from build123d import *

# Parameters (mm, degrees)
F1_DEPTH  = 8
F3_W      = 8
F3_H      = 8
F3_R      = 2.4
F4_DEPTH  = 1.7
F5_R      = 2.4
F6_DEPTH  = 1.7
F9_R      = 2.4
F10_DEPTH = 25.4


with BuildPart() as f1:
    # F0 (on Front) → F1 (new body)
    with BuildSketch(Plane.XZ):
        Polygon((-2.4, 9.6), (-4, 9.6), (-4, 0), (4, 0), (4, 9.6), (2.4, 9.6), (2.4, 11.3), (-2.4, 11.3), align=None)
    extrude(amount=F1_DEPTH)

    # F3 (on plane+point) → F4 (cut, through all)
    with BuildSketch(Plane.XY.offset(11.3)):
        with Locations((0, -4)):
            Rectangle(F3_W, F3_H)
        with Locations((0, -4)):
            Circle(F3_R, mode=Mode.SUBTRACT)
    extrude(amount=-F4_DEPTH, mode=Mode.SUBTRACT)

    # F5 (on Top) → F6 (cut)
    with BuildSketch(Plane.XY):
        with Locations((0, -4)):
            Circle(F5_R)
    extrude(amount=F6_DEPTH, mode=Mode.SUBTRACT)

    # F8: F1 across plane


with BuildPart() as f1_1:
    add(f1.part)
    add(f1.part.mirror(Plane.YZ.offset(4)))

    # F9 (on Front) → F10 (cut)
    with BuildSketch(Plane.XZ):
        with Locations((3.999, 6.4008)):
            Circle(F9_R)
    extrude(amount=F10_DEPTH, mode=Mode.SUBTRACT)


solid = f1_1.part
The listing builds one solid part. Answer for the finished solid, in the listing's coordinates (mm). A direction names the side the tool comes from. Coordinates: 2 decimals unless noted, no trailing zeros. Write each loop counter-clockwise with the first axis right and the second up, starting at its lowest first coordinate (ties: lowest second). Pieces come first, ordered by that corner, then holes. Notation, with made-up numbers: M 48,-33.5 L 101,-33.5 A22 ccw 101,-5.5 Z; hole C 61.25,3.5 d6. An arc over 180 degrees is marked long. Write each question's results on one line, items separated by ' | '.
Item 1: Consider probe 1 along Y at (x, z) = (0, 0.9); probe 2 along Z at (x, y) = (-2.75, -7); probe 3 along Z at (x, y) = (5.75, -5.25). Determine where each line is inside the solid, lowest interval first. Write a range as [from, to].
Answer below:
probe 1: [-8, -6.4], [-1.6, 0] | probe 2: [0, 9.6] | probe 3: [0, 4.76], [8.04, 9.6]
Item 2: The part is cut by section A-A on x = 8. Determine the outline of the cut face in (y, z).
Answer below:
outline: M -8,0 L -6.4,0 L -6.4,1.7 L -1.6,1.7 L -1.6,0 L 0,0 L 0,9.6 L -1.6,9.6 L -1.6,11.3 L -6.4,11.3 L -6.4,9.6 L -8,9.6 Z
Item 3: The part is cut by section B-B on z = 5.5. Determine the outline of the cut face in (x, y), and give its area (3 significant figures).
Answer below:
outline: M -4,-8 L 1.77,-8 L 1.77,0 L -4,0 Z; M 6.22,-8 L 12,-8 L 12,0 L 6.22,0 Z | area: 92.4 mm2
Item 4: Given P1, Ø1.5, axis at x = 1.5, y = -4, coming from the -Z side; P2, Ø1.5, axis at x = 5.5, y = -6, coming from the +Z side, each flat-ended and moving along its own axis, determine where each tip first touches the part or whether it passes through.
Answer below:
P1: z = 1.7 | P2: z = 9.6
Item 5: For a pull along Y with two mould halves and no side action, classify faces 1 (the face through (1.29, -1.976, 10.462)), 2 (the face through (0, -4, 11.3)), 3 (the face through (10.398, -3.894, 0.838)) as released by +Y, released by -Y, zero draft, split by the parting line, or undercut.
Answer below:
face 1: split by the parting line | face 2: zero draft | face 3: undercut
Item 6: The part is cut by section C-C on y = -4. Determine the outline of the cut face in (x, z).
Answer below:
outline: M -4,0 L -2.4,0 L -2.4,1.7 L 2.4,1.7 L 2.4,0 L 5.6,0 L 5.6,1.7 L 10.4,1.7 L 10.4,0 L 12,0 L 12,9.6 L 10.4,9.6 L 10.4,11.3 L 5.6,11.3 L 5.6,9.6 L 2.4,9.6 L 2.4,11.3 L -2.4,11.3 L -2.4,9.6 L -4,9.6 Z; hole C 4,6.4 d4.8
Item 7: Which of the six approach directions +Z, -Z, +X, -X, +Y, -Y give full straight-line access (tool end or side, diameter ignored) to faces 4 (the face through (8, -4, 11.3)), 5 (the face through (8, -4, 1.7)), 6 (the face through (4, -4, 9.6))?
Answer below:
face 4: +Z, +X, -X, +Y, -Y | face 5: -Z | face 6: +Z
Item 8: The part is cut by section D-D on z = 1.25. Determine the outline of the cut face in (x, y).
Answer below:
outline: M -4,-8 L 12,-8 L 12,0 L -4,0 Z; hole C 0,-4 d4.8; hole C 8,-4 d4.8
